CAD build for the part. Positions are in the model's coordinates, mm. A direction names the side the tool comes from. Coordinates: 2 decimals unless noted, no trailing zeros. Order: outer loops, then holes, each group sorted by start corner. A loop starts at its lowest first (then second) coordinate and runs counter-clockwise, first axis right, second up. Notation, with made-up numbers: M 88,-14.5 L 112,-14.5 A20 cw 112,24.5 Z; hole C -28.5,46.5 d3. An arc over 180 degrees is marked long. Write item = value, one per line. Start each with the question number.
```python
from build123d import *

# Parameters (mm, degrees)
SKETCH1_W            = 609.6
SKETCH1_H            = 730.25
SKETCH1_W_2          = 406.4
SKETCH1_H_2          = 527.05
BOSS_EXTRUDE1_DEPTH  = 50.8
SKETCH2_W            = 101.6
SKETCH2_H            = 50.8
BOSS_EXTRUDE2_DEPTH  = 1524
SKETCH3_W            = 304.8
SKETCH3_H            = 50.8
BOSS_EXTRUDE3_DEPTH  = 50.8
SKETCH4_W            = 101.6
SKETCH4_H            = 12.7
BOSS_EXTRUDE4_DEPTH  = 101.6
SKETCH4_2_W          = 101.6
SKETCH4_2_H          = 12.7
BOSS_EXTRUDE5_DEPTH  = 50.8
SKETCH5_W            = 609.6
SKETCH5_H            = 730.25
SKETCH5_W_2          = 406.4
SKETCH5_H_2          = 527.05
BOSS_EXTRUDE6_DEPTH  = 50.8
SKETCH7_W            = 304.8
SKETCH7_H            = 50.8
BOSS_EXTRUDE7_DEPTH  = 50.8
SKETCH8_W            = 101.6
SKETCH8_H            = 12.7
BOSS_EXTRUDE8_DEPTH  = 50.8
SKETCH8_2_W          = 101.6
SKETCH8_2_H          = 12.7
BOSS_EXTRUDE9_DEPTH  = 101.6
SKETCH9_R            = 6.35
CUT_EXTRUDE1_DEPTH   = 12.7
SKETCH10_R           = 9.525
BOSS_EXTRUDE10_DEPTH = 50.8
SKETCH10_3_W         = 76.2
SKETCH10_3_H         = 76.2
SKETCH10_3_R         = 9.525
BOSS_EXTRUDE11_DEPTH = 6.35


with BuildPart() as part:
    # Sketch1 → Boss-Extrude1 (new body)
    with BuildSketch(Plane(origin=(-762, 0, 0), x_dir=(0, 0, -1), z_dir=(1, 0, 0))):
        with Locations((0, 263.525)):
            Rectangle(SKETCH1_W, SKETCH1_H)
        with Locations((0, 263.525)):
            Rectangle(SKETCH1_W_2, SKETCH1_H_2, mode=Mode.SUBTRACT)
    extrude(amount=-BOSS_EXTRUDE1_DEPTH)

    # Sketch2 → Boss-Extrude2 (add)
    with BuildSketch(Plane(origin=(-762, 0, 0), x_dir=(0, 0, -1), z_dir=(1, 0, 0))):
        Polygon((-203.2, 50.8), (-203.2, 0), (-152.4, 0), (-152.4, -50.8), (-254, -50.8), (-254, 50.8), align=None)
        Polygon((203.2, 50.8), (203.2, 0), (152.4, 0), (152.4, -50.8), (254, -50.8), (254, 50.8), align=None)
        with Locations((-254, 501.65)):
            Rectangle(SKETCH2_W, SKETCH2_H)
        with Locations((254, 501.65)):
            Rectangle(SKETCH2_W, SKETCH2_H)
    extrude(amount=BOSS_EXTRUDE2_DEPTH)

    # Sketch3 → Boss-Extrude3 (add)
    with BuildSketch(Plane(origin=(-762, 0, 0), x_dir=(0, 0, -1), z_dir=(1, 0, 0))):
        Polygon((-152.4, -50.8), (-254, -50.8), (-254, -254), (-152.4, -254), (-152.4, -247.65), (-152.4, -196.85), align=None)
        with Locations((0, -222.25)):
            Rectangle(SKETCH3_W, SKETCH3_H)
        Polygon((152.4, -50.8), (152.4, -196.85), (152.4, -247.65), (152.4, -254), (254, -254), (254, -50.8), align=None)
        Polygon((152.4, -260.35), (-152.4, -260.35), (-152.4, -311.15), (99.92547286, -311.15), (152.4, -311.15), align=None)
        Polygon((-152.4, -254), (-254, -254), (-254, -1336.675), (-152.4, -1336.675), (-152.4, -1285.875), (-152.4, -311.15), (-152.4, -260.35), align=None)
        Polygon((254, -254), (152.4, -254), (152.4, -260.35), (152.4, -311.15), (152.4, -1285.875), (152.4, -1336.675), (254, -1336.675), align=None)
        Polygon((99.92547286, -311.15), (-152.4, -1285.875), (-99.92547286, -1285.875), (152.4, -311.15), align=None)
        Polygon((-152.4, -1285.875), (-152.4, -1336.675), (152.4, -1336.675), (152.4, -1285.875), (-99.92547286, -1285.875), align=None)
    extrude(amount=BOSS_EXTRUDE3_DEPTH)

    # Sketch4 → Boss-Extrude4 (add)
    with BuildSketch(Plane(origin=(-762, 0, 0), x_dir=(0, 0, -1), z_dir=(1, 0, 0))):
        with Locations((-203.2, -254)):
            Rectangle(SKETCH4_W, SKETCH4_H)
        with Locations((203.2, -254)):
            Rectangle(SKETCH4_W, SKETCH4_H)
    extrude(amount=BOSS_EXTRUDE4_DEPTH)

    # Sketch4_2 → Boss-Extrude5 (add)
    with BuildSketch(Plane(origin=(-762, 0, 0), x_dir=(0, 0, -1), z_dir=(1, 0, 0))):
        with Locations((-203.2, -254)):
            Rectangle(SKETCH4_2_W, SKETCH4_2_H)
        with Locations((203.2, -254)):
            Rectangle(SKETCH4_2_W, SKETCH4_2_H)
    extrude(amount=-BOSS_EXTRUDE5_DEPTH)

    # Sketch5 → Boss-Extrude6 (add)
    with BuildSketch(Plane(origin=(762, 0, 0), x_dir=(0, 0, -1), z_dir=(1, 0, 0))):
        with Locations((0, 263.525)):
            Rectangle(SKETCH5_W, SKETCH5_H)
        with Locations((0, 263.525)):
            Rectangle(SKETCH5_W_2, SKETCH5_H_2, mode=Mode.SUBTRACT)
    extrude(amount=BOSS_EXTRUDE6_DEPTH)

    # Sketch7 → Boss-Extrude7 (add)
    with BuildSketch(Plane(origin=(762, 0, 0), x_dir=(0, 0, -1), z_dir=(1, 0, 0))):
        Polygon((-152.4, -50.8), (-254, -50.8), (-254, -254), (-152.4, -254), (-152.4, -247.65), (-152.4, -196.85), align=None)
        with Locations((0, -222.25)):
            Rectangle(SKETCH7_W, SKETCH7_H)
        Polygon((152.4, -50.8), (152.4, -196.85), (152.4, -247.65), (152.4, -254), (254, -254), (254, -50.8), align=None)
        Polygon((254, -254), (152.4, -254), (152.4, -260.35), (152.4, -311.15), (152.4, -1285.875), (152.4, -1336.675), (254, -1336.675), align=None)
        Polygon((152.4, -260.35), (-152.4, -260.35), (-152.4, -311.15), (99.92547286, -311.15), (152.4, -311.15), align=None)
        Polygon((-152.4, -254), (-254, -254), (-254, -1336.675), (-152.4, -1336.675), (-152.4, -1285.875), (-152.4, -311.15), (-152.4, -260.35), align=None)
        Polygon((99.92547286, -311.15), (-152.4, -1285.875), (-99.92547286, -1285.875), (152.4, -311.15), align=None)
        Polygon((-152.4, -1285.875), (-152.4, -1336.675), (152.4, -1336.675), (152.4, -1285.875), (-99.92547286, -1285.875), align=None)
    extrude(amount=-BOSS_EXTRUDE7_DEPTH)

    # Sketch8 → Boss-Extrude8 (add)
    with BuildSketch(Plane(origin=(762, 0, 0), x_dir=(0, 0, -1), z_dir=(1, 0, 0))):
        with Locations((-203.2, -254)):
            Rectangle(SKETCH8_W, SKETCH8_H)
        with Locations((203.2, -254)):
            Rectangle(SKETCH8_W, SKETCH8_H)
    extrude(amount=BOSS_EXTRUDE8_DEPTH)

    # Sketch8_2 → Boss-Extrude9 (add)
    with BuildSketch(Plane(origin=(762, 0, 0), x_dir=(0, 0, -1), z_dir=(1, 0, 0))):
        with Locations((-203.2, -254)):
            Rectangle(SKETCH8_2_W, SKETCH8_2_H)
        with Locations((203.2, -254)):
            Rectangle(SKETCH8_2_W, SKETCH8_2_H)
    extrude(amount=-BOSS_EXTRUDE9_DEPTH)

    # Sketch9 → Cut-Extrude1 (cut)
    with BuildSketch(Plane(origin=(0, -247.65, 0), x_dir=(1, 0, 0), z_dir=(0, 1, 0))):
        with Locations(Location((-787.4, 177.8, 0), (0, 0, 270))):
            Circle(SKETCH9_R)
        with Locations(Location((-787.4, 228.6, 0), (0, 0, 270))):
            Circle(SKETCH9_R)
        with Locations(Location((-685.8, 228.6, 0), (0, 0, 270))):
            Circle(SKETCH9_R)
        with Locations(Location((-685.8, 177.8, 0), (0, 0, 270))):
            Circle(SKETCH9_R)
        with Locations(Location((-787.4, -177.8, 0), (0, 0, 270))):
            Circle(SKETCH9_R)
        with Locations(Location((-787.4, -228.6, 0), (0, 0, 270))):
            Circle(SKETCH9_R)
        with Locations(Location((-685.8, -177.8, 0), (0, 0, 270))):
            Circle(SKETCH9_R)
        with Locations(Location((-685.8, -228.6, 0), (0, 0, 270))):
            Circle(SKETCH9_R)
        with Locations(Location((685.8, -177.8, 0), (0, 0, 270))):
            Circle(SKETCH9_R)
        with Locations(Location((685.8, -228.6, 0), (0, 0, 270))):
            Circle(SKETCH9_R)
        with Locations(Location((787.4, -177.8, 0), (0, 0, 270))):
            Circle(SKETCH9_R)
        with Locations(Location((787.4, -228.6, 0), (0, 0, 270))):
            Circle(SKETCH9_R)
        with Locations(Location((685.8, 228.6, 0), (0, 0, 270))):
            Circle(SKETCH9_R)
        with Locations(Location((685.8, 177.8, 0), (0, 0, 270))):
            Circle(SKETCH9_R)
        with Locations(Location((787.4, 228.6, 0), (0, 0, 270))):
            Circle(SKETCH9_R)
        with Locations(Location((787.4, 177.8, 0), (0, 0, 270))):
            Circle(SKETCH9_R)
    extrude(amount=-CUT_EXTRUDE1_DEPTH, mode=Mode.SUBTRACT)

    # Sketch10 → Boss-Extrude10 (add)
    with BuildSketch(Plane(origin=(0, -1387.475, 0), x_dir=(-1, 0, 0), z_dir=(0, -1, 0))):
        with Locations(Location((736.6, -203.2, 0), (0, 0, 90))):
            Circle(SKETCH10_R)
        with Locations(Location((736.6, 203.2, 0), (0, 0, 90))):
            Circle(SKETCH10_R)
        with Locations(Location((-736.6, -203.2, 0), (0, 0, 90))):
            Circle(SKETCH10_R)
        with Locations(Location((-736.6, 203.2, 0), (0, 0, 90))):
            Circle(SKETCH10_R)
    extrude(amount=-BOSS_EXTRUDE10_DEPTH)

    # Sketch10_3 → Boss-Extrude11 (add)
    # profile 1 of 4: a face of its own
    with BuildSketch(Plane(origin=(0, -1387.475, 0), x_dir=(-1, 0, 0), z_dir=(0, -1, 0))):
        with Locations((-736.6, -203.2)):
            Rectangle(SKETCH10_3_W, SKETCH10_3_H)
        with Locations(Location((-736.6, -203.2, 0), (0, 0, 90))):
            Circle(SKETCH10_3_R, mode=Mode.SUBTRACT)
    # profile 2 of 4: a face of its own
    with BuildSketch(Plane(origin=(0, -1387.475, 0), x_dir=(-1, 0, 0), z_dir=(0, -1, 0))):
        with Locations((736.6, -203.2)):
            Rectangle(SKETCH10_3_W, SKETCH10_3_H)
        with Locations(Location((736.6, -203.2, 0), (0, 0, 90))):
            Circle(SKETCH10_3_R, mode=Mode.SUBTRACT)
    # profile 3 of 4: a face of its own
    with BuildSketch(Plane(origin=(0, -1387.475, 0), x_dir=(-1, 0, 0), z_dir=(0, -1, 0))):
        with Locations((-736.6, 203.2)):
            Rectangle(SKETCH10_3_W, SKETCH10_3_H)
        with Locations(Location((-736.6, 203.2, 0), (0, 0, 90))):
            Circle(SKETCH10_3_R, mode=Mode.SUBTRACT)
    # profile 4 of 4: a face of its own
    with BuildSketch(Plane(origin=(0, -1387.475, 0), x_dir=(-1, 0, 0), z_dir=(0, -1, 0))):
        with Locations((736.6, 203.2)):
            Rectangle(SKETCH10_3_W, SKETCH10_3_H)
        with Locations(Location((736.6, 203.2, 0), (0, 0, 90))):
            Circle(SKETCH10_3_R, mode=Mode.SUBTRACT)
    extrude(amount=-BOSS_EXTRUDE11_DEPTH)


solid = part.part
```
1. Slice it at C-C (y = -986). Write the cut outline in (x, z).
2. 3-axis set-ups, long thin cutter, end or side, ignore diameter. For faces 1 (the flat face through (-728, -1381.125, 211)), 2 (the flat face through (-737, -792, -152.4)), 3 (the flat face through (-56, -30, -254)), 4 (the flat face through (-762, -791, 4)), 5 (the flat face through (-686, -247.65, 204)): which of +Z, -Z, +X, -X, +Y, -Y reach the whole face in a straight line?
3. Mould opens along Y. For faces 6 (the flat face through (737, -311.15, 28)), 7 (the flat face through (-787, 628.65, 4)), 8 (the flat face through (-736, -1387.475, 203)) say: released by +Y, released by -Y, zero draft, split by the parting line, or undercut.
4. Flat gauge pins, fed straight in: pin 1 (14.5 mm diameter, centred on x = 685.8, z = 228.6, fed in from +Y); pin 2 (3 mm diameter, centred on y = -1384.5, z = 187, fed in from +X); pin 3 (15 mm diameter, centred on x = -786, z = -93, fed in from -Y). Where does each tip first touch, or does it go through?
5. Slice it at D-D (z = -1). Give the number of separate pieces and of enclosed holes in the cut face, plus the area to 3 significant figures.
6. Probe L1, parallel to X at y = -257, z = 228.6; L2, parallel to Z at x = -685.8, y = -252.5; L3, parallel to Y at x = 678.5, z = 212.5. List the from-to ranges inside material, lowest first.
7. Slice it at B-B (y = 289.5). Write the cut outline in (x, z).
8. Slice it at A-A (x = -425). Write the cut outline in (y, z).
Calculated:
q1.outline = M -762,-254 L -711.2,-254 L -711.2,-152.4 L -762,-152.4 Z; M -762,22.3 L -711.2,22.3 L -711.2,74.77 L -762,74.77 Z; M -762,152.4 L -711.2,152.4 L -711.2,254 L -762,254 Z; M 711.2,-254 L 762,-254 L 762,-152.4 L 711.2,-152.4 Z; M 711.2,22.3 L 762,22.3 L 762,74.77 L 711.2,74.77 Z; M 711.2,152.4 L 762,152.4 L 762,254 L 711.2,254 Z
q2.face_1 = none
q2.face_2 = +X, -X
q2.face_3 = -Z, -Y
q2.face_4 = +Z, -Z, -X
q2.face_5 = +Z, -Z
q3.face_6 = undercut
q3.face_7 = released by +Y
q3.face_8 = released by -Y
q4.pin_1 = 527.05
q4.pin_2 = 774.7
q4.pin_3 = -101.6
q5.separate_pieces = 12
q5.enclosed_holes = 0
q5.area = 56,700 mm²
q6.L1 = -812.8 to -793.75, -781.05 to -692.15, -679.45 to -660.4, 660.4 to 679.45, 692.15 to 781.05, 793.75 to 812.8
q6.L2 = -254 to -234.95, -222.25 to -184.15, -171.45 to -152.4, 152.4 to 171.45, 184.15 to 222.25, 234.95 to 254
q6.L3 = -260.35 to -247.65, -50.8 to 50.8, 476.25 to 527.05
q7.outline = M -812.8,-304.8 L -762,-304.8 L -762,-203.2 L -812.8,-203.2 Z; M -812.8,203.2 L -762,203.2 L -762,304.8 L -812.8,304.8 Z; M 762,-304.8 L 812.8,-304.8 L 812.8,-203.2 L 762,-203.2 Z; M 762,203.2 L 812.8,203.2 L 812.8,304.8 L 762,304.8 Z
q8.outline = M -50.8,-254 L 50.8,-254 L 50.8,-203.2 L 0,-203.2 L 0,-152.4 L -50.8,-152.4 Z; M -50.8,152.4 L 0,152.4 L 0,203.2 L 50.8,203.2 L 50.8,254 L -50.8,254 Z; M 476.25,-304.8 L 527.05,-304.8 L 527.05,-203.2 L 476.25,-203.2 Z; M 476.25,203.2 L 527.05,203.2 L 527.05,304.8 L 476.25,304.8 Z
